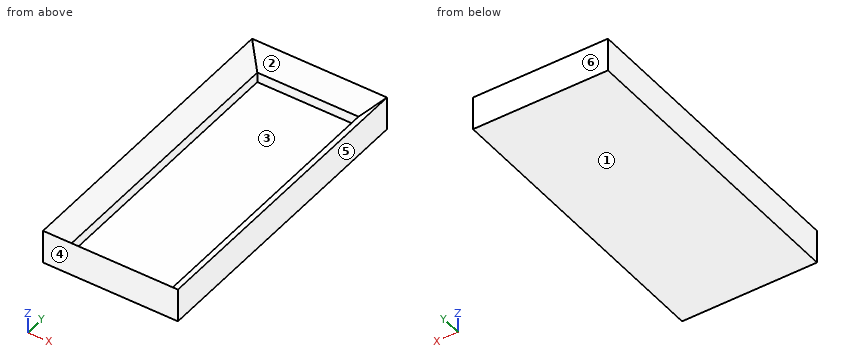
```python
from build123d import *

# Parameters (mm, degrees)
F0_W     = 40
F0_H     = 90
F0_W_2   = 30
F0_H_2   = 80
F1_DEPTH = 10
F2_DEPTH = 2
F3_SIZE  = 4.99999


# Not quite as in the source:
# - a fillet or chamfer is up to 0.001 mm smaller than in the source, because OpenCascade refuses the exact size


with BuildPart() as f1:
    # F0 (on Top) → F1 (new body)
    with BuildSketch(Plane.XY):
        with Locations((1.4284082502, 37.2216339977)):
            Rectangle(F0_W, F0_H)
        with Locations((1.4284082502, 37.2216339977)):
            Rectangle(F0_W_2, F0_H_2, mode=Mode.SUBTRACT)
    extrude(amount=F1_DEPTH)

    # F0 (on Top) → F2 (join)
    with BuildSketch(Plane.XY):
        with Locations((1.4284082502, 37.2216339977)):
            Rectangle(F0_W_2, F0_H_2)
    extrude(amount=F2_DEPTH)

    # F3 (size 5 in the source; OpenCascade refuses exactly that, so slightly less here)
    f3_edges = [f1.edges().sort_by_distance(p)[0] for p in [
        (16.428408, 37.221634, 10),
        (1.428408, 77.221634, 10),
        (-13.571592, 37.221634, 10),
        (1.428408, -2.778366, 10),
    ]]
    chamfer(f3_edges, length=F3_SIZE)


solid = f1.part
```
Geometry check sheet. Reference: the model listing, model coordinates, mm. Face numbers are marked on the shaded views. A direction names the side the tool comes from. Coordinates: 2 decimals unless noted, no trailing zeros. Order: outer loops, then holes, each group sorted by start corner. A loop starts at its lowest first (then second) coordinate and runs counter-clockwise, first axis right, second up. Notation, with made-up numbers: M 41.5,-18 L 70.5,-18 A22 ccw 70.5,5 Z; hole C -35.75,36 d8. An arc over 180 degrees is marked long. Answer as a JSON object with one key per item and string values.
Q1. Cross-section at C-C on z = 7.75. Record the cut outline in (x, y), and give its area (3 significant figures).
Results are:
{"outline": "M -18.57,-7.78 L 21.43,-7.78 L 21.43,82.22 L -18.57,82.22 Z; hole M -16.32,-5.53 L 19.18,-5.53 L 19.18,79.97 L -16.32,79.97 Z", "area": "565 mm²"}
Q2. Scan lines: line 1 (X direction, y = 71, z = 4); line 2 (Y direction, x = 11.5, z = 4.5); line 3 (Z direction, x = -7.5, y = 10). Record each from-to range of solid material in increasing order.
Results are:
{"line 1": "x = -18.57 to -13.57, 16.43 to 21.43", "line 2": "y = -7.78 to -2.78, 77.22 to 82.22", "line 3": "z = 0 to 2"}
Q3. Release check for a two-part mould opening along Y. For the marked faces 3, 4, 5 and 6 record: released by +Y, released by -Y, zero draft, split by the parting line, or undercut.
Results are:
{"face 3": "undercut", "face 4": "released by -Y", "face 5": "zero draft", "face 6": "released by +Y"}
Q4. Tool access check on the marked faces 1 and 2. Record the directions out of +Z, -Z, +X, -X, +Y, -Y that give a thin tool (end or side, any length) a straight path to the whole face; none if there is none.
Results are:
{"face 1": "-Z, +X, -X, +Y, -Y", "face 2": "+Z"}
Q5. Depth check by flat-ended pin: pin 1 Ø8 at (x, y) = (-9, 67) entering from +Z. Enter the tip coordinate at first touch or a pass-through.
Results are:
{"pin 1": "stops at z = 2"}
